from build123d import *

# Parameters (mm, degrees)
Y_KSEKLIK_EKSTR_ZYON1_DEPTH     = 60
KES_EKSTR_ZYON1_DEPTH           = 60
IZIM3_R                         = 1.5
KES_EKSTR_ZYON2_DEPTH           = 60
RADYUS1_R                       = 15
RADYUS2_R                       = 5
IZIM4_R                         = 1.75
IZIM4_W                         = 40
IZIM4_H                         = 20
KES_EKSTR_ZYON3_DEPTH           = 60
Y_KSEKLIK_EKSTR_ZYON2_START     = 4
IZIM5_R                         = 1.75
IZIM5_R_2                       = 1.5
IZIM5_W                         = 40
IZIM5_H                         = 20
Y_KSEKLIK_EKSTR_ZYON2_DEPTH     = 4
PAH1_SIZE                       = 4
RADYUS3_R                       = 4
KES_EKSTR_ZYON4_DEPTH           = 4
Y_KSEKLIK_EKSTR_ZYON3_START     = -4
Y_KSEKLIK_EKSTR_ZYON3_OUTLINE_W = 5
Y_KSEKLIK_EKSTR_ZYON3_OUTLINE_H = 19
Y_KSEKLIK_EKSTR_ZYON3_DEPTH     = 4
IZIM8_R                         = 15
Y_KSEKLIK_EKSTR_ZYON4_DEPTH     = 2
Y_KSEKLIK_EKSTR_ZYON5_START     = -8
Y_KSEKLIK_EKSTR_ZYON5_DEPTH     = 8
IZIM10_R                        = 1.75
KES_EKSTR_ZYON5_DEPTH           = 10
Y_KSEKLIK_EKSTR_ZYON6_START     = -8
Y_KSEKLIK_EKSTR_ZYON6_DEPTH     = 8
KES_EKSTR_ZYON6_START           = -10
IZIM12_R                        = 1.75
KES_EKSTR_ZYON6_DEPTH           = 10
IZIM13_R                        = 1.75
KES_EKSTR_ZYON7_DEPTH           = 10
RADYUS4_R                       = 10


# Read off the part's stored shape, not the designer's step: Yükseklik-Ekstrüzyon3, Yükseklik-Ekstrüzyon5, Yükseklik-Ekstrüzyon6
with BuildPart() as part:
    # Çizim1 → Yükseklik-Ekstrüzyon1 (new body)
    with BuildSketch(Plane.XY):
        with BuildLine():
            Line((0, 0), (80, 0))
            Line((80, 0), (80, 30))
            ThreePointArc((80, 30), (81.171572875, 32.828427125), (84, 34))
            Line((84, 34), (224, 34))
            Line((224, 34), (224, 38))
            Line((224, 38), (78, 38))
            ThreePointArc((78, 38), (75.171572875, 36.828427125), (74, 34))
            Line((74, 34), (74, 4))
            Line((74, 4), (0, 4))
            Line((0, 4), (0, 0))
        make_face()
    extrude(amount=Y_KSEKLIK_EKSTR_ZYON1_DEPTH)

    # Çizim2 → Kes-Ekstrüzyon1 (cut)
    with BuildSketch(Plane.ZY.offset(-74)):
        with BuildLine():
            Line((16, 29), (20, 29))
            ThreePointArc((20, 29), (25.656854249, 26.656854249), (28, 21))
            Line((28, 21), (28, 12.482548154))
            ThreePointArc((28, 12.482548154), (26.687092043, 9.312907957), (23.517451846, 8))
            Line((23.517451846, 8), (12.482548154, 8))
            ThreePointArc((12.482548154, 8), (9.312907957, 9.312907957), (8, 12.482548154))
            Line((8, 12.482548154), (8, 21))
            ThreePointArc((8, 21), (10.343145751, 26.656854249), (16, 29))
        make_face()
        with BuildLine():
            Line((32, 21), (32, 12.482548154))
            ThreePointArc((32, 12.482548154), (33.312907957, 9.312907957), (36.482548154, 8))
            Line((36.482548154, 8), (47.517451846, 8))
            ThreePointArc((47.517451846, 8), (50.687092043, 9.312907957), (52, 12.482548154))
            Line((52, 12.482548154), (52, 21))
            ThreePointArc((52, 21), (49.656854249, 26.656854249), (44, 29))
            Line((44, 29), (40, 29))
            ThreePointArc((40, 29), (34.343145751, 26.656854249), (32, 21))
        make_face()
    extrude(amount=-KES_EKSTR_ZYON1_DEPTH, mode=Mode.SUBTRACT)

    # Çizim3 → Kes-Ekstrüzyon2 (cut)
    with BuildSketch(Plane(origin=(0, 4, 0), x_dir=(1, 0, 0), z_dir=(0, 1, 0))):
        with Locations(Location((5, -15.5, 0), (0, 0, 180))):
            Circle(IZIM3_R)
        with Locations(Location((5, -44.5, 0), (0, 0, 180))):
            Circle(IZIM3_R)
        with Locations(Location((65, -15.5, 0), (0, 0, 180))):
            Circle(IZIM3_R)
        with Locations(Location((65, -44.5, 0), (0, 0, 180))):
            Circle(IZIM3_R)
    extrude(amount=-KES_EKSTR_ZYON2_DEPTH, mode=Mode.SUBTRACT)

    # Radyus1
    radyus1_edges = [part.edges().sort_by_distance(p)[0] for p in [
        (0, 2, 0),
        (0, 2, 60),
    ]]
    fillet(radyus1_edges, radius=RADYUS1_R)

    # Radyus2
    radyus2_edges = [part.edges().sort_by_distance(p)[0] for p in [
        (80, 0, 30),
    ]]
    fillet(radyus2_edges, radius=RADYUS2_R)

    # Çizim4 → Kes-Ekstrüzyon3 (cut)
    with BuildSketch(Plane(origin=(0, 4, 0), x_dir=(1, 0, 0), z_dir=(0, 1, 0))):
        with Locations(Location((21.11, -25, 0), (0, 0, 180))):
            Circle(IZIM4_R)
        with Locations(Location((21.11, -35, 0), (0, 0, 180))):
            Circle(IZIM4_R)
        with Locations(Location((69.11, -25, 0), (0, 0, 180))):
            Circle(IZIM4_R)
        with Locations(Location((69.11, -35, 0), (0, 0, 180))):
            Circle(IZIM4_R)
        with Locations((45.11, -30)):
            Rectangle(IZIM4_W, IZIM4_H)
    extrude(amount=-KES_EKSTR_ZYON3_DEPTH, mode=Mode.SUBTRACT)

    # Çizim5 → Yükseklik-Ekstrüzyon2 (add)
    with BuildSketch(Plane(origin=(0, 4, 0), x_dir=(1, 0, 0), z_dir=(0, 1, 0)).offset(Y_KSEKLIK_EKSTR_ZYON2_START)):
        with BuildLine():
            Line((24.11, -13), (74, -13))
            Line((74, -13), (74, -47))
            Line((74, -47), (24.11, -47))
            ThreePointArc((24.11, -47), (19.867359313, -45.242640687), (18.11, -41))
            Line((18.11, -41), (18.11, -19))
            ThreePointArc((18.11, -19), (19.867359313, -14.757359313), (24.11, -13))
        make_face()
        with Locations(Location((21.11, -25, 0), (0, 0, 180))):
            Circle(IZIM5_R, mode=Mode.SUBTRACT)
        with Locations(Location((21.11, -35, 0), (0, 0, 180))):
            Circle(IZIM5_R, mode=Mode.SUBTRACT)
        with Locations(Location((65, -44.5, 0), (0, 0, 180))):
            Circle(IZIM5_R_2, mode=Mode.SUBTRACT)
        with Locations(Location((69.11, -25, 0), (0, 0, 180))):
            Circle(IZIM5_R, mode=Mode.SUBTRACT)
        with Locations(Location((69.11, -35, 0), (0, 0, 180))):
            Circle(IZIM5_R, mode=Mode.SUBTRACT)
        with Locations(Location((65, -15.5, 0), (0, 0, 180))):
            Circle(IZIM5_R_2, mode=Mode.SUBTRACT)
        with Locations((45.11, -30)):
            Rectangle(IZIM5_W, IZIM5_H, mode=Mode.SUBTRACT)
    extrude(amount=-Y_KSEKLIK_EKSTR_ZYON2_DEPTH)

    # Pah1
    pah1_edges = [part.edges().sort_by_distance(p)[0] for p in [
        (49.055, 4, 13),
        (19.867359313, 4, 14.757359313),
        (18.11, 4, 30),
        (19.867359313, 4, 45.242640687),
        (49.055, 4, 47),
    ]]
    chamfer(pah1_edges, length=PAH1_SIZE - 0.0001)  # a hair under: the kernel refuses the full size

    # Radyus3
    radyus3_edges = [part.edges().sort_by_distance(p)[0] for p in [
        (74, 4, 55.49995),
        (74, 4, 4.50005),
    ]]
    fillet(radyus3_edges, radius=RADYUS3_R - 0.0001)  # a hair under: the kernel refuses the full size

    # Çizim6 → Kes-Ekstrüzyon4 (cut)
    with BuildSketch(Plane(origin=(0, 38, 0), x_dir=(1, 0, 0), z_dir=(0, 1, 0))):
        with BuildLine():
            Line((204, -52), (98, -52))
            ThreePointArc((98, -52), (90.928932188, -49.071067812), (88, -42))
            Line((88, -42), (88, -33))
            Line((88, -33), (214, -33))
            Line((214, -33), (214, -42))
            ThreePointArc((214, -42), (211.071067812, -49.071067812), (204, -52))
        make_face()
        with BuildLine():
            Line((204, -8), (98, -8))
            ThreePointArc((98, -8), (90.928932188, -10.928932188), (88, -18))
            Line((88, -18), (88, -27))
            Line((88, -27), (214, -27))
            Line((214, -27), (214, -18))
            ThreePointArc((214, -18), (211.071067812, -10.928932188), (204, -8))
        make_face()
    extrude(amount=-KES_EKSTR_ZYON4_DEPTH, mode=Mode.SUBTRACT)

    # Yükseklik-Ekstrüzyon3 outline → Yükseklik-Ekstrüzyon3 (add)
    with BuildSketch(Plane(origin=(0, 38, 0), x_dir=(1, 0, 0), z_dir=(0, 1, 0)).offset(Y_KSEKLIK_EKSTR_ZYON3_START)):
        with Locations((173.5, -42.5)):
            Rectangle(Y_KSEKLIK_EKSTR_ZYON3_OUTLINE_W, Y_KSEKLIK_EKSTR_ZYON3_OUTLINE_H)
        with Locations((128.5, -42.5)):
            Rectangle(Y_KSEKLIK_EKSTR_ZYON3_OUTLINE_W, Y_KSEKLIK_EKSTR_ZYON3_OUTLINE_H)
        with Locations((173.5, -17.5)):
            Rectangle(Y_KSEKLIK_EKSTR_ZYON3_OUTLINE_W, Y_KSEKLIK_EKSTR_ZYON3_OUTLINE_H)
        with Locations((128.5, -17.5)):
            Rectangle(Y_KSEKLIK_EKSTR_ZYON3_OUTLINE_W, Y_KSEKLIK_EKSTR_ZYON3_OUTLINE_H)
    extrude(amount=Y_KSEKLIK_EKSTR_ZYON3_DEPTH)

    # Çizim8 → Yükseklik-Ekstrüzyon4 (add)
    with BuildSketch(Plane(origin=(0, 38, 0), x_dir=(1, 0, 0), z_dir=(0, 1, 0))):
        with Locations((128.5, -30)):
            Circle(IZIM8_R)
    extrude(amount=-Y_KSEKLIK_EKSTR_ZYON4_DEPTH)

    # Yükseklik-Ekstrüzyon5 outline → Yükseklik-Ekstrüzyon5 (add)
    with BuildSketch(Plane.XY.offset(60).offset(Y_KSEKLIK_EKSTR_ZYON5_START)):
        with BuildLine():
            Line((179.263932023, 38), (183.736067977, 38))
            ThreePointArc((183.736067977, 38), (181.5, 39), (179.263932023, 38))
        make_face()
        with BuildLine():
            Line((183.736067977, 34), (179.263932023, 34))
            ThreePointArc((179.263932023, 34), (181.5, 33), (183.736067977, 34))
        make_face()
    extrude(amount=Y_KSEKLIK_EKSTR_ZYON5_DEPTH)

    # Çizim10 → Kes-Ekstrüzyon5 (cut)
    with BuildSketch(Plane.XY.offset(60)):
        with Locations((181.5, 36)):
            Circle(IZIM10_R)
    extrude(amount=-KES_EKSTR_ZYON5_DEPTH, mode=Mode.SUBTRACT)

    # Yükseklik-Ekstrüzyon6 outline → Yükseklik-Ekstrüzyon6 (add)
    with BuildSketch(Plane(origin=(0, 0, 0), x_dir=(-1, 0, 0), z_dir=(0, 0, -1)).offset(Y_KSEKLIK_EKSTR_ZYON6_START)):
        with BuildLine():
            Line((-183.736067977, 38), (-179.263932023, 38))
            ThreePointArc((-179.263932023, 38), (-181.5, 39), (-183.736067977, 38))
        make_face()
        with BuildLine():
            Line((-179.263932023, 34), (-183.736067977, 34))
            ThreePointArc((-183.736067977, 34), (-181.5, 33), (-179.263932023, 34))
        make_face()
    extrude(amount=Y_KSEKLIK_EKSTR_ZYON6_DEPTH)

    # Çizim12 → Kes-Ekstrüzyon6 (cut)
    with BuildSketch(Plane(origin=(0, 0, 0), x_dir=(-1, 0, 0), z_dir=(0, 0, -1)).offset(KES_EKSTR_ZYON6_START)):
        with Locations(Location((-181.5, 36, 0), (0, 0, 180))):
            Circle(IZIM12_R)
    extrude(amount=KES_EKSTR_ZYON6_DEPTH, mode=Mode.SUBTRACT)

    # Çizim13 → Kes-Ekstrüzyon7 (cut)
    with BuildSketch(Plane(origin=(0, 38, 0), x_dir=(1, 0, 0), z_dir=(0, 1, 0))):
        with Locations(Location((219, -30, 0), (0, 0, 180))):
            Circle(IZIM13_R)
    extrude(amount=-KES_EKSTR_ZYON7_DEPTH, mode=Mode.SUBTRACT)

    # Radyus4
    radyus4_edges = [part.edges().sort_by_distance(p)[0] for p in [
        (224, 36, 0),
        (224, 36, 60),
    ]]
    fillet(radyus4_edges, radius=RADYUS4_R)


solid = part.part
Can you work these out from the model? Positions are in its coordinate system, mm. A direction names the side the tool comes from. Coordinates: 2 decimals unless noted, no trailing zeros. Answer as a JSON object with one key per item and string values. Group by question number.
Q1. We'd pull the mould along X, two halves only. Please class faces 6 (the face through (117.984, 37.014, 40.697)), 7 (the face through (0, 2, 30)), 8 (the face through (77, 29, 42)): +X half, -X half, draft (parallel to the pull), parting line (faces both ways), or undercut.
Q2. Will these pins go through, and if not, where does the flat tip stop? P1, Ø3.5, axis at x = 117, z = 38, coming from the -Y side; P2, Ø3, axis at y = 37, z = 38, coming from the -X side; P3, Ø2.5, axis at y = 4, z = 25.5, coming from the +X side; P4, Ø10, axis at x = 86.5, y = 11, coming from the +Z side.
Q3. On a 3-axis mill with a long thin cutter (end or side, diameter ignored), from which of +Z, -Z, +X, -X, +Y, -Y can I reach the whole of each face in a straight line? I mean faces 1 (the face through (16.08, 5.97, 30.15)), 2 (the face through (80, 17, 30)), 3 (the face through (136, 36, 38)), 4 (the face through (88, 36, 22)), 5 (the face through (77, 29, 18)). Say none if no direction works.
Q4. I need wall thicknesses on line 1 (Z direction, x = 65, y = 3); line 2 (Z direction, x = 5, y = 1.9); line 3 (Y direction, x = 158, z = 57). Which ranges of each line are inside material? Lowest first, please. Write a range as from..to.
Determined:
{
 "1": {"face 6": "undercut", "face 7": "-X half", "face 8": "draft"},
 "2": {"P1": "stops at y = 36", "P2": "stops at x = 74.29", "P3": "stops at x = 80", "P4": "passes through"},
 "3": {"face 1": "+Z, -Z, -X, +Y", "face 2": "+Z, -Z, +X, -Y", "face 3": "-Y", "face 4": "+Y, -Y", "face 5": "+X, -X"},
 "4": {"line 1": "z = 0..14, 17..20, 40..43, 46..60", "line 2": "z = 3.82..14, 17..43, 46..56.18", "line 3": "y = 34..38"}
}
